from build123d import *

# Parameters (mm, degrees)
F0_R     = 10
F1_DEPTH = 90
F2_R     = 8
F3_R     = 5
F4_R     = 3.5
F5_DEPTH = 45
F6_R     = 1.5
F7_DEPTH = 10.001


with BuildPart() as f1:
    # F0 (on Top) → F1 (new body)
    with BuildSketch(Plane.XY):
        Circle(F0_R)
    extrude(amount=F1_DEPTH)

    # F2
    f2_edges = [f1.edges().sort_by_distance(p)[0] for p in [
        (-10, 0, 0),
    ]]
    fillet(f2_edges, radius=F2_R)

    # F3
    f3_edges = [f1.edges().sort_by_distance(p)[0] for p in [
        (-10, 0, 90),
    ]]
    fillet(f3_edges, radius=F3_R)

    # F4 (on face) → F5 (cut)
    with BuildSketch(Plane.XY.offset(90)):
        Circle(F4_R)
    extrude(amount=-F5_DEPTH, mode=Mode.SUBTRACT)

    # F6 (on Front) → F7 (cut, through all)
    with BuildSketch(Plane.XZ):
        with Locations((0, 75)):
            Circle(F6_R)
    extrude(amount=-F7_DEPTH, mode=Mode.SUBTRACT)


solid = f1.part
Work out the finished part from the listing and answer in its coordinate system (mm). A direction names the side the tool comes from. Give positions to 0.01 mm unless a question says otherwise; leave off trailing zeros. Loops run counter-clockwise (first coordinate to the right, second up) from the corner with the lowest first, then second, coordinate; pieces in that order, holes last. Notation, with made-up numbers: (17, -37) - (33, -37) arc R24 cw to (33, -17) - close; hole circle Ø2 at (33, 35.25). An arc over 180 degrees is marked (long way). Answer in a Markdown table with one row per item. Add a question column.
Q1. The part is cut by section C-C (z = 75). Determine the outline of the cut face in (x, y).
Q2. Consider line 1 along Y through (x, z) = (0, 79); line 2 along X through (y, z) = (7, 75); line 3 along Z through (x, y) = (1, 9). Determine where each line is inside the solid, lowest interval first.
Q3. The part is cut by section A-A (z = 15). Determine the outline of the cut face in (x, y).
Q4. The part is cut by section B-B (z = 49.5). Determine the outline of the cut face in (x, y).
Q5. Each of these flat-tipped pins is pushed along its axis until it touches: P1, Ø8, axis at x = 1.5, z = 71, coming from the +Y side; P2, Ø3.5, axis at x = -1.5, y = 0, coming from the +Z side; P3, Ø2.5, axis at x = 0, z = 75, coming from the +Y side; P4, Ø1.5, axis at x = 0.5, y = 6.5, coming from the +Z side. Where does it stop, or does it pass through?
Q6. A tool of negligible diameter and unlimited length cuts with its end or side. For faces 4 (the flat face through (2.2, -3.3, 90)), 5 (the cylindrical face through (3.233, -1.341, 67.815)), from which of +Z, -Z, +X, -X, +Y, -Y can it reach the whole face along a straight path? Write none if from no direction.
Q7. Determine the mould class of faces 1 (the flat face through (0, 0, 45)), 2 (the cylindrical face through (0.69, 6.53, 73.67)), 3 (the cylindrical face through (-2.17, -9.76, 45.96)) for opening direction Y: released by +Y, released by -Y, zero draft, split by the parting line, or undercut.
Solution:
| question | item | result |
|---|---|---|
| 1 | outline | (-1.5, 3.16) - (-1.5, 9.89) arc R10 ccw (long way) to (1.5, 9.89) - (1.5, 3.16) arc R3.5 cw (long way) to start |
| 2 | line 1 | y = -10 to -3.5, 3.5 to 10 |
| 2 | line 2 | x = -7.14 to -1.5, 1.5 to 7.14 |
| 2 | line 3 | z = 4.23 to 73.88, 76.12 to 87.92 |
| 3 | outline | circle Ø20 at (0, 0) |
| 4 | outline | circle Ø20 at (0, 0); hole circle Ø7 at (0, 0) |
| 5 | P1 | stops at y = 10 |
| 5 | P2 | stops at z = 45 |
| 5 | P3 | stops at y = -3.27 |
| 5 | P4 | stops at z = 89.94 |
| 6 | face 4 | +Z, +X, -X, +Y, -Y |
| 6 | face 5 | +Z |
| 7 | face 1 | undercut |
| 7 | face 2 | zero draft |
| 7 | face 3 | split by the parting line |
